```python
from build123d import *

# Parameters (mm, degrees)
SKETCH2_R                    = 3.282457618
BASE_FLANGE1_DEPTH           = 3.175
EDGE_FLANGE1_STRIP_W         = 19.05
EDGE_FLANGE1_STRIP_H         = 3.175
EDGE_FLANGE1_STRIP_CUT_DEPTH = 37
EDGE_FLANGE1_DEPTH           = 37
SKETCH6_R                    = 3.15
CUT_EXTRUDE1_DEPTH           = 10


# Sheet-metal steps are written as plain solids
with BuildPart() as part:
    # Sketch2 → Base-Flange1 (new body)
    with BuildSketch(Plane(origin=(0, 0, 0), x_dir=(0, 0, -1), z_dir=(1, 0, 0))):
        with BuildLine():
            Line((50.159054546, 37), (50.159054546, 0))
            Line((50.159054546, 0), (67.597909272, 0))
            ThreePointArc((67.597909272, 0), (69.925870777, 0.575003364), (71.718398003, 2.167761907))
            Line((71.718398003, 2.167761907), (95.660507303, 37))
            Line((95.660507303, 37), (50.159054546, 37))
        make_face()
        with Locations((73.009854993, 28.405566411)):
            Circle(SKETCH2_R, mode=Mode.SUBTRACT)
        with Locations((66.344990455, 9.222294526)):
            Circle(SKETCH2_R, mode=Mode.SUBTRACT)
    extrude(amount=-BASE_FLANGE1_DEPTH)

    # Edge-Flange1 strip (across the edge) → Edge-Flange1 strip cut (cut)
    with BuildSketch(Plane(origin=(0, 37, -50.159054546), x_dir=(0, 0, -1), z_dir=(0, -1, 0))):
        with Locations((-3.175, -1.5875)):
            Rectangle(EDGE_FLANGE1_STRIP_W, EDGE_FLANGE1_STRIP_H)
    extrude(amount=EDGE_FLANGE1_STRIP_CUT_DEPTH, mode=Mode.SUBTRACT)

    # Edge-Flange1 section (across the edge) → Edge-Flange1 (add)
    with BuildSketch(Plane(origin=(0, 37, -50.159054546), x_dir=(0, 0, -1), z_dir=(0, -1, 0))):
        with BuildLine():
            Line((0, 3.175), (0, 12.825))
            Line((0, 12.825), (3.175, 12.825))
            Line((3.175, 12.825), (3.175, 3.175))
            ThreePointArc((3.175, 3.175), (4.10493597, 0.92993597), (6.35, 0))
            Line((6.35, 0), (6.35, -3.175))
            ThreePointArc((6.35, -3.175), (1.859871939, -1.315128061), (0, 3.175))
        make_face()
    extrude(amount=EDGE_FLANGE1_DEPTH)

    # Sketch6 → Cut-Extrude1 (cut)
    with BuildSketch(Plane(origin=(0, 0, -53.334054546), x_dir=(-1, 0, 0), z_dir=(0, 0, -1))):
        with Locations((-8, 18.5)):
            Circle(SKETCH6_R)
    extrude(amount=-CUT_EXTRUDE1_DEPTH, mode=Mode.SUBTRACT)


solid = part.part
```
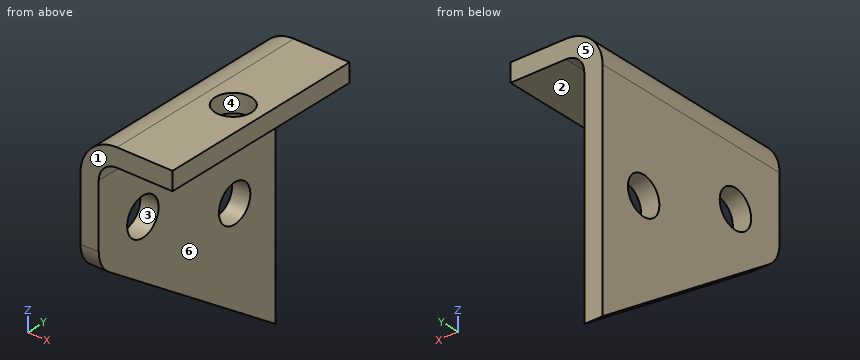
Geometry: final body of the model. Coordinates: model frame, mm. Face numbers are marked on the shaded views. A direction names the side the tool comes from. Round coordinates to 2 decimals unless told otherwise and drop trailing zeros. Order: outer loops, then holes, each group sorted by start corner. A loop starts at its lowest first (then second) coordinate and runs counter-clockwise, first axis right, second up. Notation, with made-up numbers: (80.5, 64) -> (112.5, 64) arc R16 cw to (112.5, 94) -> close; hole circle Ø11 at (46, 6.5). An arc over 180 degrees is marked (long way). Use one line per item in the form item = value. Start each with the question number.
1. Draft query along Y for the marked faces 3, 4, 5 and 6. Return one class per face: pulls with the +Y half, pulls with the -Y half, needs draft (parallel to the pull), parting line crosses it, or undercut.
2. Cut plane D-D (z = -57.5). Return the cut outline in (x, y) (3 decimals), then the cut area to 3 significant figures.
3. Cut plane A-A (x = 8). Return the cut outline in (y, z), then the cut area to 3 significant figures.
4. Line query: probe 1 along Y at (x, z) = (8, -52.25); probe 2 along X at (y, z) = (14, -74) (3 decimals); probe 3 along Z at (x, y) = (9.5, 7). Output: solid intervals per line, ascending.
5. Cut plane B-B (y = 18.5). Return the cut outline in (x, z) (3 decimals), then the cut area to 3 significant figures.
6. Pin query (flat end, axial travel): pin 1 Ø4 at (x, z) = (3.5, -80) entering from -Y; pin 2 Ø5 at (x, y) = (10, 20) entering from -Z; pin 3 Ø18.5 at (y, z) = (19.5, -86) entering from +X; pin 4 Ø2 at (y, z) = (10.5, -55) entering from +X. Return the tip coordinate at first contact, or that it passes through.
7. Cut plane C-C (x = -1). Return the cut outline in (y, z) (1 decimal), then the cut area to 3 significant figures.
8. Reachability of the marked faces 1 and 2 from +Z, -Z, +X, -X, +Y, -Y: full face, straight path, thin tool, end or side. Return the list, or none.
Solution:
q1.face_3 = undercut
q1.face_4 = undercut
q1.face_5 = pulls with the +Y half
q1.face_6 = needs draft
q2.outline = (-3.175, 0) -> (0, 0) -> (0, 37) -> (-3.175, 37) -> close
q2.area = 117 mm^2
q3.outline = (0, -53.33) -> (15.35, -53.33) -> (15.35, -50.16) -> (0, -50.16) -> close; (21.65, -53.33) -> (37, -53.33) -> (37, -50.16) -> (21.65, -50.16) -> close
q3.area = 97.5 mm^2
q4.probe_1 = 0 to 15.35, 21.65 to 37
q4.probe_2 = -3.175 to 0
q4.probe_3 = -53.33 to -50.16
q5.outline = (-3.175, -82.944) -> (0, -82.944) -> (0, -56.509) arc R3.175 cw to (3.175, -53.334) -> (4.85, -53.334) -> (4.85, -50.159) -> (3.175, -50.159) arc R6.35 ccw to (-3.175, -56.509) -> close; (11.15, -53.334) -> (12.825, -53.334) -> (12.825, -50.159) -> (11.15, -50.159) -> close
q5.area = 118 mm^2
q6.pin_1 = through
q6.pin_2 = -53.33
q6.pin_3 = 0
q6.pin_4 = 1.23
q7.outline = (0, -67.6) arc R5 ccw to (2.2, -71.7) -> (37, -95.7) -> (37, -51.7) -> (0, -51.7) -> close; hole circle Ø6.6 at (9.2, -66.3); hole circle Ø6.6 at (28.4, -73)
q7.area = 1,090 mm^2
q8.face_1 = +Z, -Z, +X, -X, -Y
q8.face_2 = -Z, +X, +Y, -Y
